Source: CAD feature listing. Evaluate the final solid. Frame: model axes, mm. Face numbers are marked on the shaded views. A direction names the side the tool comes from. Coordinates: 2 decimals unless noted, no trailing zeros. Write each loop counter-clockwise with the first axis right and the second up, starting at its lowest first coordinate (ties: lowest second). Pieces come first, ordered by that corner, then holes. Notation, with made-up numbers: (-17, -14) - (9, -14) arc R18 ccw to (9, 11) - close; hole circle Ø2 at (0, 63). An arc over 180 degrees is marked (long way). One line per item, written item: value.
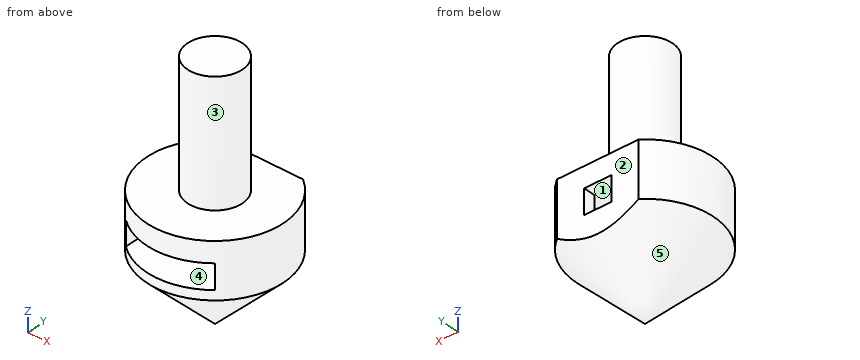
from build123d import *

# Parameters (mm, degrees)
SKETCH008_W     = 10
SKETCH008_H     = 1.5
POCKET004_DEPTH = 9.001
POCKET005_DEPTH = 1.8


with BuildPart() as part:
    # Sketch007 → Revolution001 (revolve)
    with BuildSketch(Plane.XZ):
        Polygon((0, 0), (0, -18), (5, -13), (5, -9), (2, -9), (2, 0), align=None)
    revolve(axis=Axis((0, 0, 0), (0, 0, 1)))

    # Sketch008 (on Face3 of Revolution001) → Pocket004 (cut, through all)
    with BuildSketch(Plane(origin=(0, 0, -9), x_dir=(-1, 0, 0), z_dir=(0, 0, 1))):
        with Locations((0, -4.75)):
            Rectangle(SKETCH008_W, SKETCH008_H)
    extrude(amount=-POCKET004_DEPTH, mode=Mode.SUBTRACT)

    # Sketch009 (on Face5 of Pocket004) → Pocket005 (cut)
    with BuildSketch(Plane(origin=(0, 0, -10.5), x_dir=(-1, 0, 0), z_dir=(0, 0, 1))):
        with BuildLine():
            ThreePointArc((-3.275, 0), (-2.64581, -1.930107), (-1, -3.118593))
            Line((-1, -3.118593), (-1, -6.5))
            Line((-1, -6.5), (1, -6.5))
            Line((1, -6.5), (1, -3.113342))
            ThreePointArc((1, -3.113342), (2.642243, -1.926512), (3.27, 0))
            Line((3.27, 6.5), (3.27, 0))
            Line((-3.275, 6.5), (3.27, 6.5))
            Line((-3.275, 0), (-3.275, 6.5))
        make_face()
    extrude(amount=-POCKET005_DEPTH, mode=Mode.SUBTRACT)


solid = part.part
1) Reachability of the marked faces 1 and 2 from +Z, -Z, +X, -X, +Y, -Y: full face, straight path, thin tool, end or side. Return the list, or none.
Values found:
face 1: -Y
face 2: +Z, -Z, +X, -X, +Y
2) Material intervals for line 1 (Z direction, x = -1.75, y = -4.25); line 2 (Z direction, x = 1.5, y = -2); line 3 (X direction, y = 0.75, z = -16.5), sorted ascending.
Values found:
line 1: -13.4 to -12.3, -10.5 to -9
line 2: -15.5 to -12.3, -10.5 to -9
line 3: -1.3 to 1.3
3) Section query B-B on z = -10.25. Output: boundary loops of the cut face in (x, y), then the cut area to 3 significant figures.
Values found:
outline: (-3, 4) arc R5 ccw (long way) to (3, 4) - close
area: 74.5 mm2
4) Contact query for flat-ended pins moving along their axis: P1, Ø4, axis at x = -4, y = -2.5, coming from the +Z side; P2, Ø0.5, axis at y = -2, z = -11.5, coming from the +X side; P3, Ø0.7, axis at y = 3.5, z = -11, coming from the +X side; P4, Ø3.5, axis at x = -1, y = -1.5, coming from the +Z side. Output: stop coordinate, or through.
Values found:
P1: z = -9
P2: x = 4.68
P3: x = 3.88
P4: z = 0
5) Section query C-C on z = -3.5. Output: boundary loops of the cut face in (x, y).
Values found:
outline: circle Ø4 at (0, 0)
6) Draft query along Z for the marked faces 3, 4 and 5. Return one class per face: released by +Z, released by -Z, zero draft, split by the parting line, or undercut.
Values found:
face 3: zero draft
face 4: undercut
face 5: released by -Z
7) Section query A-A on z = -14.5. Output: boundary loops of the cut face in (x, y), then the cut area to 3 significant figures.
Values found:
outline: circle Ø7 at (0, 0)
area: 38.5 mm2
